Autodesk Inventor part; units mm, degrees
ref_plane "YZ Plane" through (0, 0, 0) normal (1, 0, 0) x (0, 1, 0)
ref_plane "XZ Plane" through (0, 0, 0) normal (0, 1, 0) x (-1, 0, 0)
ref_plane "XY Plane" through (0, 0, 0) normal (0, 0, 1) x (1, 0, 0)
sketch "スケッチ1" plane through (0, 0, 0) normal (0, 0, 1) x (1, 0, 0)
  line L0 (-3.5, 3.5) -> (3.5, 3.5)
  line L1 (3.5, 3.5) -> (3.5, -3.5)
  line L2 (3.5, -3.5) -> (-3.5, -3.5)
  line L3 (-3.5, -3.5) -> (-3.5, 3.5)
  line L4 (-3.5, 3.5) -> (3.5, -3.5) construction
  line L5 (3.5, 3.5) -> (-3.5, -3.5) construction
  point P0 (0, 0)
  dimension "d0" = 7
  dimension "d2" = 7
extrude "押し出し1" add sketch "スケッチ1" along normal blind 5
sketch "スケッチ2" plane through (3.5, -3.5, 0) normal (1, 0, 0) x (0, 0, -1)
  line L0 (-5, 0) -> (-5, 7)
  line L1 (0, 0) -> (-5, 0)
  point P0 (0, 3.5)
  point P1 (-2.5, 3.5)
  dimension "d5" = 2.5
  dimension "d6" = 3.5
hole "穴1" at (3.5, 0, 2.5) direction (-1, 0, 0) diameter 2.459 end through all
sketch "スケッチ3" plane through (0, 0, 5) normal (0, 0, 1) x (1, 0, 0)
  line L0 (3.5, 3.5) -> (-3.5, 3.5)
  line L1 (-3.5, 3.5) -> (-3.5, -3.5)
  line L2 (-3.5, -3.5) -> (3.5, -3.5)
  line L3 (3.5, -3.5) -> (3.5, 3.5)
  circle A0 centre (0, 0) radius 3.5
  point P0 (0, 0)
extrude "押し出し2" cut sketch "スケッチ3" against normal blind 5 contours L3 A0 L0 | A0 L1 L0 | L3 L2 A0 | A0 L2 L1
sketch "スケッチ4" plane through (0, 0, 5) normal (0, 0, 1) x (1, 0, 0)
  circle A0 centre (0, 0) radius 3.5
  circle A1 centre (0, 0) radius 1.5
  dimension "d16" = 3
hole "穴2" at (0, 0, 5) at (0, 0, 5) direction (0, 0, -1) diameter 3 end through all
properties part number "sttopa" material "アルミニウム 2014-T4"
Verification items for the finished model (mm, model axes). Round coordinates to 2 decimals unless told otherwise and drop trailing zeros. Order: outer loops, then holes, each group sorted by start corner. A loop starts at its lowest first (then second) coordinate and runs counter-clockwise, first axis right, second up. Notation, with made-up numbers: (77.5, -36.75) -> (99.5, -36.75) arc R11 ccw to (99.5, -20.75) -> close; hole circle Ø9 at (-29, 15.5). An arc over 180 degrees is marked (long way). Put each result on its own line as item: value. Start each with the question number.
(1) Depth check by flat-ended pin: pin 1 Ø2 at (y, z) = (0, 2.5) entering from -X; pin 2 Ø1 at (x, z) = (1.5, 2.5) entering from +Y. Enter the tip coordinate at first touch or a pass-through.
(2) Section check D-D (z = 0.8). Enter the section's corners in (x, y).
(3) Section check A-A (x = 0). Enter the section's corners in (y, z), then the cut area to 3 significant figures.
(4) Section check B-B (y = 0). Enter the section's corners in (x, z).
(5) Material ranges on line 1 along Y through (x, z) = (0, 2.35); line 2 along Z through (x, y) = (2, 0); line 3 along Y through (x, z) = (2.5, 2.65), recorded low to high.
(6) Draft check along X on faces 1 (the face through (1.615, -3.105, 2.535)), 2 (the face through (0.575, -1.386, 2.465)), 3 (the face through (-2.2, -0.05, 3.73)). Enter one of: +X half, -X half, draft (parallel to the pull), parting line (faces both ways), or undercut.
(7) Section check C-C (z = 3.55). Enter the section's corners in (x, y).
Completed:
1. pin 1: passes through
1. pin 2: stops at y = 3.35
2. outline: circle Ø7 at (0, 0); hole circle Ø3 at (0, 0)
3. outline: (-3.5, 0) -> (-1.5, 0) -> (-1.5, 5) -> (-3.5, 5) -> close; (1.5, 0) -> (3.5, 0) -> (3.5, 5) -> (1.5, 5) -> close
3. area: 20.0 mm2
4. outline: (-3.5, 0) -> (-1.5, 0) -> (-1.5, 1.27) -> (-3.5, 1.27) -> close; (-3.5, 3.73) -> (-1.5, 3.73) -> (-1.5, 5) -> (-3.5, 5) -> close; (1.5, 0) -> (3.5, 0) -> (3.5, 1.27) -> (1.5, 1.27) -> close; (1.5, 3.73) -> (3.5, 3.73) -> (3.5, 5) -> (1.5, 5) -> close
5. line 1: y = -3.5 to -1.5, 1.5 to 3.5
5. line 2: z = 0 to 1.27, 3.73 to 5
5. line 3: y = -2.45 to -1.22, 1.22 to 2.45
6. face 1: parting line
6. face 2: undercut
6. face 3: draft
7. outline: (-3.44, -0.64) arc R3.5 ccw to (3.44, -0.64) -> (1.36, -0.64) arc R1.5 cw to (-1.36, -0.64) -> close; (-3.44, 0.64) -> (-1.36, 0.64) arc R1.5 cw to (1.36, 0.64) -> (3.44, 0.64) arc R3.5 ccw to start
